from build123d import *

# Parameters (mm, degrees)
SKETCH1_R           = 5.830122714
BOSS_EXTRUDE1_DEPTH = 50.8
FILLET1_R           = 6.35


with BuildPart() as part:
    # Sketch1 → Boss-Extrude1 (new body)
    with BuildSketch(Plane.XY):
        with BuildLine():
            Line((-31.75, -31.75), (73.130794165, -31.75))
            ThreePointArc((73.130794165, -31.75), (91.531681156, -17.630502809), (82.655794165, 3.797783942))
            Line((82.655794165, 3.797783942), (-3.175, 53.352216058))
            ThreePointArc((-3.175, 53.352216058), (-22.225, 53.352216058), (-31.75, 36.854432116))
            Line((-31.75, 36.854432116), (-31.75, -31.75))
        make_face()
        Circle(SKETCH1_R, mode=Mode.SUBTRACT)
    extrude(amount=BOSS_EXTRUDE1_DEPTH)

    # Fillet1
    fillet1_edges = [part.edges().sort_by_distance(p)[0] for p in [
        (91.531681156, -17.630502809, 50.8),
        (39.740397082, 28.575, 50.8),
        (-22.225, 53.352216058, 50.8),
        (-31.75, 2.552216058, 50.8),
        (-22.225, 53.352216058, 0),
        (39.740397082, 28.575, 0),
        (91.531681156, -17.630502809, 0),
        (20.690397082, -31.75, 0),
        (-31.75, 2.552216058, 0),
        (20.690397082, -31.75, 50.8),
    ]]
    fillet(fillet1_edges, radius=FILLET1_R)


solid = part.part
Input: part model. Units: mm. Frame: model coordinates. Coordinates: 2 decimals unless noted, no trailing zeros. Order: outer loops, then holes, each group sorted by start corner. A loop starts at its lowest first (then second) coordinate and runs counter-clockwise, first axis right, second up.
1. Cut plane A-A, the plane z = 27. Return loops of the section in (x, y) (3 decimals).
Checked values:
outline: (-31.75, -31.75) - (73.131, -31.75) arc R19.05 ccw to (82.656, 3.798) - (-3.175, 53.352) arc R19.05 ccw to (-31.75, 36.854) - close; hole circle Ø11.66 at (0, 0)
2. Contact query for flat-ended pins moving along their axis: P1, Ø4, axis at y = -22.5, z = 12, coming from the +X side; P2, Ø13.5, axis at x = 0, y = 0, coming from the +Z side; P3, Ø10, axis at x = 28.5, z = 19.5, coming from the +Y side; P4, Ø1.5, axis at y = -6, z = 22.5, coming from the +X side. Output: stop coordinate, or through.
Checked values:
P1: stops at x = 90.51
P2: stops at z = 50.8
P3: stops at y = 37.95
P4: stops at x = 91.23
3. Ray query, line 1 along Y through (x, z) = (0, 38); line 2 along Y through (x, z) = (-1, 39.5); line 3 along X through (y, z) = (1, 47.5). Return the intervals inside material, ascending.
Checked values:
line 1: y = -31.75 to -5.83, 5.83 to 51.52
line 2: y = -31.75 to -5.74, 5.74 to 52.1
line 3: x = -30.97 to -5.74, 5.74 to 85.22
